from build123d import *

# Parameters (mm, degrees)
EXTRUDE_1_DEPTH     = 104
SKETCH_2_R          = 2
SKETCH_2_R_2        = 2.5
SKETCH_2_W          = 6.5
SKETCH_2_H          = 80
CUT_EXTRUDE_1_DEPTH = 132.346869015


with BuildPart() as part:
    # 草图1 → 凸台-拉伸1 (new body)
    with BuildSketch(Plane(origin=(0, 0, 0), x_dir=(0, 0, -1), z_dir=(1, 0, 0))):
        Polygon((0, 0), (80, 0), (80, 6), (6, 6), (0, 6), align=None)
    extrude(amount=EXTRUDE_1_DEPTH)

    # 草图2 → 切除-拉伸1 (cut, through all)
    with BuildSketch(Plane(origin=(0, 6, 0), x_dir=(1, 0, 0), z_dir=(0, 1, 0))):
        with Locations(Location((43, 11, 0), (0, 0, 270))):
            Circle(SKETCH_2_R)
        with Locations(Location((43, 35, 0), (0, 0, 270))):
            Circle(SKETCH_2_R)
        with Locations(Location((42, 48, 0), (0, 0, 270))):
            Circle(SKETCH_2_R)
        with Locations(Location((42, 72, 0), (0, 0, 270))):
            Circle(SKETCH_2_R)
        with Locations(Location((62, 72, 0), (0, 0, 90))):
            Circle(SKETCH_2_R)
        with Locations(Location((62, 48, 0), (0, 0, 90))):
            Circle(SKETCH_2_R)
        with Locations(Location((61, 35, 0), (0, 0, 90))):
            Circle(SKETCH_2_R)
        with Locations(Location((61, 11, 0), (0, 0, 90))):
            Circle(SKETCH_2_R)
        with Locations(Location((57.5, 23, 0), (0, 0, 270))):
            Circle(SKETCH_2_R_2)
        with Locations(Location((89.5, 23, 0), (0, 0, 270))):
            Circle(SKETCH_2_R_2)
        with Locations(Location((46.5, 23, 0), (0, 0, 90))):
            Circle(SKETCH_2_R_2)
        with Locations(Location((14.5, 23, 0), (0, 0, 90))):
            Circle(SKETCH_2_R_2)
        with Locations(Location((73, 60, 0), (0, 0, 270))):
            Circle(SKETCH_2_R)
        with Locations(Location((31, 60, 0), (0, 0, 270))):
            Circle(SKETCH_2_R)
        with Locations((100.75, 40)):
            Rectangle(SKETCH_2_W, SKETCH_2_H)
        with Locations((3.25, 40)):
            Rectangle(SKETCH_2_W, SKETCH_2_H)
    extrude(amount=-CUT_EXTRUDE_1_DEPTH, mode=Mode.SUBTRACT)


solid = part.part
Geometry: final body of the model. Coordinates: model frame, mm. Give positions to 0.01 mm unless a question says otherwise; leave off trailing zeros. Order: outer loops, then holes, each group sorted by start corner. A loop starts at its lowest first (then second) coordinate and runs counter-clockwise, first axis right, second up. Notation, with made-up numbers: (66.25, -37.5) -> (124.25, -37.5) arc R16 cw to (124.25, -32.5) -> close; hole circle Ø11 at (-21.5, -39). An arc over 180 degrees is marked (long way). Put each result on its own line as item: value.
Q1. Section B-B, the plane x = 88. Return loops of the section in (y, z), then the cut area to 3 significant figures.
Here are the results:
outline: (0, -80) -> (6, -80) -> (6, -25) -> (0, -25) -> close; (0, -21) -> (6, -21) -> (6, 0) -> (0, 0) -> close
area: 456 mm^2
Q2. Section D-D, the plane x = 61. Return loops of the section in (y, z).
Here are the results:
outline: (0, -80) -> (6, -80) -> (6, -73.73) -> (0, -73.73) -> close; (0, -70.27) -> (6, -70.27) -> (6, -49.73) -> (0, -49.73) -> close; (0, -46.27) -> (6, -46.27) -> (6, -37) -> (0, -37) -> close; (0, -33) -> (6, -33) -> (6, -13) -> (0, -13) -> close; (0, -9) -> (6, -9) -> (6, 0) -> (0, 0) -> close
Q3. Section C-C, the plane y = 1.35. Count the separate pieces of the cut face and the enclosed holes in it, then the cut area to 3 significant figures.
Here are the results:
separate pieces: 1
enclosed holes: 14
area: 7,080 mm^2
Q4. Pin query (flat end, axial travel): pin 1 (3.5 mm diameter, centred on x = 42, z = -48, fed in from +Y). Return the tip coordinate at first contact, or that it passes through.
Here are the results:
pin 1: passes through
Q5. Section A-A, the plane z = -72. Return loops of the section in (x, y).
Here are the results:
outline: (6.5, 0) -> (40, 0) -> (40, 6) -> (6.5, 6) -> close; (44, 0) -> (60, 0) -> (60, 6) -> (44, 6) -> close; (64, 0) -> (97.5, 0) -> (97.5, 6) -> (64, 6) -> close
Q6. Material intervals for L1, parallel to X at y = 1.85, z = -23; L2, parallel to X at y = 1.6, z = -48; L3, parallel to X at y = 4.2, z = -60, sorted ascending.
Here are the results:
L1: x = 6.5 to 12, 17 to 44, 49 to 55, 60 to 87, 92 to 97.5
L2: x = 6.5 to 40, 44 to 60, 64 to 97.5
L3: x = 6.5 to 29, 33 to 71, 75 to 97.5
Q7. Draft query along Z for faces 1 (the face through (40.226, 3.042, -71.077)), 2 (the face through (51, 6, -41)), 3 (the face through (41.226, 3.042, -34.077)), 4 (the face through (51, 3, 0)). Return one class per face: released by +Z, released by -Z, zero draft, split by the parting line, or undercut.
Here are the results:
face 1: undercut
face 2: zero draft
face 3: undercut
face 4: released by +Z
